```python
from build123d import *

# Parameters (mm, degrees)
SKETCH2_W          = 0.8
SKETCH2_H          = 11.5
CUT_EXTRUDE1_DEPTH = 48.41307844
CIRPATTERN1_COUNT  = 4


with BuildPart() as part:
    # Sketch1 → Revolve-Thin1 (revolve)
    with BuildSketch(Plane(origin=(0, 0, 0), x_dir=(0, 0, -1), z_dir=(1, 0, 0)), mode=Mode.PRIVATE) as revolve_thin1_sk:
        with BuildLine():
            Line((0, 7.5), (-28.725975148, 16.990434754))
            ThreePointArc((-28.725975148, 16.990434754), (-31.822634352, 17.745995734), (-35, 18))
            Line((-35, 18), (-40, 18))
            Line((-40, 18), (-40, 17.5))
            Line((-40, 17.5), (-35, 17.5))
            ThreePointArc((-35, 17.5), (-31.902068494, 17.252345841), (-28.882825769, 16.515673885))
            Line((-28.882825769, 16.515673885), (-0.156850621, 7.025239131))
            Line((-0.156850621, 7.025239131), (0, 7.5))
        make_face()
    revolve(revolve_thin1_sk.sketch.rotate(Axis((0, 0, 0), (0, 0, 1)), 90), axis=Axis((0, 0, 0), (0, 0, 1)))

    # Sketch2 → Cut-Extrude1 (cut, through all)
    with BuildSketch(Plane(origin=(0, 0, 0), x_dir=(1, 0, 0), z_dir=(0, 1, 0))):
        with Locations((0, -34.25)):
            Rectangle(SKETCH2_W, SKETCH2_H)
    cut_extrude1 = extrude(amount=-CUT_EXTRUDE1_DEPTH, mode=Mode.SUBTRACT)

    # CirPattern1: Cut-Extrude1 ×4 about axis
    cirpattern1_axis = Axis((0, 0, 0), (0, 0, 1))
    for i in range(1, CIRPATTERN1_COUNT):
        add(cut_extrude1.rotate(cirpattern1_axis, i * 360 / CIRPATTERN1_COUNT), mode=Mode.SUBTRACT)


solid = part.part
```
Geometry: final body of the model. Coordinates: model frame, mm. A direction names the side the tool comes from. Round coordinates to 2 decimals unless told otherwise and drop trailing zeros. Order: outer loops, then holes, each group sorted by start corner. A loop starts at its lowest first (then second) coordinate and runs counter-clockwise, first axis right, second up. Notation, with made-up numbers: (6, -36.5) -> (18, -36.5) arc R22 cw to (18, -12.5) -> close; hole circle Ø5 at (67, -14.5). An arc over 180 degrees is marked (long way). Use CSV: the item, a comma, the result in double quotes. Start each with the question number.
1) Section C-C (z = 25). Return the cut outline in (x, y), and give its area (3 significant figures).
2) Set-up query: faces 1 (the face through (12.51, 12.24, 37.46)), 2 (the face through (-12, 13, 40)). Return all of +Z, -Z, +X, -X, +Y, -Y with unobstructed straight access to the full face (end or side cutting, diameter ignored); none if empty.
3) Draft query along X for faces 3 (the face through (-17.8, -0.4, 34.3)), 4 (the face through (12.24, -12.51, 37.46)), 5 (the face through (-12.591, 12.863, 37.535)). Return one class per face: +X half, -X half, draft (parallel to the pull), parting line (faces both ways), or undercut.
4) First-contact query: pin 1 Ø0.6 at (x, y) = (17, 0) entering from +Z; pin 2 Ø1.8 at (y, z) = (-17, 33) entering from +X; pin 3 Ø1.5 at (y, z) = (-5, 8.5) entering from -X; pin 4 Ø1 at (x, y) = (-5, -2.5) entering from -Z. Flat tips, straight axial feed; report the tip coordinate or a pass-through.
5) Material intervals for line 1 along X through (y, z) = (3.5, 32.5); line 2 along X through (y, z) = (-8.5, 36.5); line 3 along Y through (x, z) = (3, 6), sorted ascending. Write a range as from..to.
6) Section A-A (z = 5.5). Return the cut outline in (x, y), and give its area (3 significant figures).
Returned:
1,outline,"circle Ø31.52 at (0, 0); hole circle Ø30.47 at (0, 0)"
1,area,"51.3 mm²"
2,face 1,"+Z"
2,face 2,"+Z, +X, -X, +Y, -Y"
3,face 3,"draft"
3,face 4,"undercut"
3,face 5,"-X half"
4,pin 1,"stops at z = 28.5"
4,pin 2,"stops at x = 7.83"
4,pin 3,"stops at x = -9.49"
4,pin 4,"passes through"
5,line 1,"x = -17.5..-16.98, 16.98..17.5"
5,line 2,"x = -15.87..-15.3, 15.3..15.87"
5,line 3,"y = -9..-8.44, 8.44..9"
6,outline,"circle Ø18.63 at (0, 0); hole circle Ø17.58 at (0, 0)"
6,area,"30.0 mm²"
